The model under review builds one solid part; all positions refer to its coordinate system, in mm. A direction names the side the tool comes from. Round coordinates to 2 decimals unless told otherwise and drop trailing zeros. Write each loop counter-clockwise with the first axis right and the second up, starting at its lowest first coordinate (ties: lowest second). Pieces come first, ordered by that corner, then holes. Notation, with made-up numbers: (18, -30.5) - (56, -30.5) arc R26 ccw to (56, -7.5) - close; hole circle Ø5 at (15, -25.5). An arc over 180 degrees is marked (long way). One line per question, with ' | ' between items. Start each with the question number.
```python
from build123d import *

# Parameters (mm, degrees)
F1_DEPTH = 7
F2_D     = 4


with BuildPart() as f1:
    # F0 (on Front) → F1 (new body)
    with BuildSketch(Plane.XZ):
        with BuildLine():
            Line((4.413146, 27.5), (4.413146, -27.5))
            Line((4.413146, -27.5), (-9.336854, -27.5))
            ThreePointArc((-9.336854, -27.5), (-15.586854, -33.75), (-9.336854, -40))
            Line((-9.336854, -40), (16.913146, -40))
            Line((16.913146, -40), (16.913146, 40))
            Line((16.913146, 40), (-9.336854, 40))
            ThreePointArc((-9.336854, 40), (-15.586854, 33.75), (-9.336854, 27.5))
            Line((-9.336854, 27.5), (4.413146, 27.5))
        make_face()
    extrude(amount=F1_DEPTH)

    # F2 (through all)
    with Locations(Plane(origin=(0, 0, 0), x_dir=(1, 0, 0), z_dir=(0, 1, 0))):
        with Locations((-9.336854, 33.75), (10.663146, 33.75), (-9.336854, -33.75), (10.663146, -33.75)):
            Hole(F2_D / 2)


solid = f1.part
```
1. Add section A-A, the plane x = 1. Write out the cut boundary in (y, z).
2. Add section B-B, the plane z = 33.75. Write out the cut boundary in (x, y).
3. Add section D-D, the plane z = 20.5. Write out the cut boundary in (x, y), then the cut area to 3 significant figures.
4. Machinability: for faces 1 (the face through (4, -3, 40)), 2 (the face through (4.413, -3, 0)), which of the approach directions +Z, -Z, +X, -X, +Y, -Y give a long, thin tool a straight path to every point of the face, cutting with its end or side? Answer none if there is none.
5. Clearance check with flat-ended pins moving along their axes: P1, Ø12, axis at x = -6.5, z = -15, coming from the +Y side; P2, Ø2, axis at y = -3, z = -5, coming from the -X side. State where each tip first meets the part, or that it passes through.
6. Add section C-C, the plane y = -4. Write out the cut boundary in (x, z).
7. Wall thickness on line 1 along X through (y, z) = (-2.25, -33.75); line 2 along Z through (x, y) = (10.5, -3.5); line 3 along Z through (x, y) = (-10, -3.25): over which ranges is each line inside the solid? List them lowest first. Write a range as [from, to].
8. The part is to be moulded in two halves that separate along X. For faces 3 (the face through (11.1, -3.5, -31.8)), 4 (the face through (8, 0, 1)), 5 (the face through (-15.585, -3.451, -33.613)), say which applies: pulls with the +X half, pulls with the -X half, needs draft (parallel to the pull), parting line crosses it, or undercut.
Geometry check:
1) outline: (-7, -40) - (0, -40) - (0, -27.5) - (-7, -27.5) - close; (-7, 27.5) - (0, 27.5) - (0, 40) - (-7, 40) - close
2) outline: (-15.59, -7) - (-11.34, -7) - (-11.34, 0) - (-15.59, 0) - close; (-7.34, -7) - (8.66, -7) - (8.66, 0) - (-7.34, 0) - close; (12.66, -7) - (16.91, -7) - (16.91, 0) - (12.66, 0) - close
3) outline: (4.41, -7) - (16.91, -7) - (16.91, 0) - (4.41, 0) - close | area: 87.5 mm2
4) face 1: +Z, +X, -X, +Y, -Y | face 2: -X, +Y, -Y
5) P1: passes through | P2: stops at x = 4.41
6) outline: (-9.34, -40) - (16.91, -40) - (16.91, 40) - (-9.34, 40) arc R6.25 ccw to (-9.34, 27.5) - (4.41, 27.5) - (4.41, -27.5) - (-9.34, -27.5) arc R6.25 ccw to start; hole circle Ø4 at (-9.34, -33.75); hole circle Ø4 at (-9.34, 33.75); hole circle Ø4 at (10.66, -33.75); hole circle Ø4 at (10.66, 33.75)
7) line 1: x = [-15.59, -11.34], [-7.34, 8.66], [12.66, 16.91] | line 2: z = [-40, -35.74], [-31.76, 31.76], [35.74, 40] | line 3: z = [-39.96, -35.64], [-31.86, -27.54], [27.54, 31.86], [35.64, 39.96]
8) face 3: undercut | face 4: needs draft | face 5: pulls with the -X half
